Input: part model. Units: mm. Frame: model coordinates. A direction names the side the tool comes from. Coordinates: 2 decimals unless noted, no trailing zeros. Loops run counter-clockwise (first coordinate to the right, second up) from the corner with the lowest first, then second, coordinate; pieces in that order, holes last. Notation, with made-up numbers: (-11.5, -4) -> (29.5, -4) arc R14 ccw to (29.5, 9) -> close; hole circle Ø11 at (-16.5, -4). An arc over 180 degrees is marked (long way). Answer as a JSON object with one key per item and string values.
from build123d import *

# Parameters (mm, degrees)
SKETCH1_R           = 2
SKETCH1_R_2         = 4
SKETCH1_R_3         = 1.95
SKETCH1_R_4         = 1.5
BOSS_EXTRUDE1_DEPTH = 3


with BuildPart() as part:
    # Sketch1 → Boss-Extrude1 (new body)
    with BuildSketch(Plane.XY.offset(-5.551615438)):
        with BuildLine():
            Line((-25.464626351, 10.13731735), (25.464626351, 10.13731735))
            ThreePointArc((25.464626351, 10.13731735), (26.878839913, 9.551530913), (27.464626351, 8.13731735))
            Line((27.464626351, 8.13731735), (27.464626351, -6.86268265))
            ThreePointArc((27.464626351, -6.86268265), (26.878839913, -8.276896212), (25.464626351, -8.86268265))
            Line((25.464626351, -8.86268265), (10, -8.86268265))
            Line((10, -8.86268265), (10, -24.66268265))
            Line((10, -24.66268265), (7.1, -24.66268265))
            Line((7.1, -24.66268265), (7.1, -20.66268265))
            Line((7.1, -20.66268265), (8.4, -20.66268265))
            Line((8.4, -20.66268265), (8.4, -17.86268265))
            Line((8.4, -17.86268265), (7.1, -17.86268265))
            Line((7.1, -17.86268265), (7.1, -6.86268265))
            Line((7.1, -6.86268265), (2.9, -6.86268265))
            Line((2.9, -6.86268265), (2.9, -17.86268265))
            Line((2.9, -17.86268265), (1.6, -17.86268265))
            Line((1.6, -17.86268265), (1.6, -20.66268265))
            Line((1.6, -20.66268265), (2.9, -20.66268265))
            Line((2.9, -20.66268265), (2.9, -24.66268265))
            Line((2.9, -24.66268265), (0, -24.66268265))
            Line((0, -24.66268265), (-2.9, -24.66268265))
            Line((-2.9, -24.66268265), (-2.9, -20.66268265))
            Line((-2.9, -20.66268265), (-1.6, -20.66268265))
            Line((-1.6, -20.66268265), (-1.6, -17.86268265))
            Line((-1.6, -17.86268265), (-2.9, -17.86268265))
            Line((-2.9, -17.86268265), (-2.9, -6.86268265))
            Line((-2.9, -6.86268265), (-7.1, -6.86268265))
            Line((-7.1, -6.86268265), (-7.1, -17.86268265))
            Line((-7.1, -17.86268265), (-8.4, -17.86268265))
            Line((-8.4, -17.86268265), (-8.4, -20.66268265))
            Line((-8.4, -20.66268265), (-7.1, -20.66268265))
            Line((-7.1, -20.66268265), (-7.1, -24.66268265))
            Line((-7.1, -24.66268265), (-10, -24.66268265))
            Line((-10, -24.66268265), (-10, -8.86268265))
            Line((-10, -8.86268265), (-25.464626351, -8.86268265))
            ThreePointArc((-25.464626351, -8.86268265), (-26.878839913, -8.276896212), (-27.464626351, -6.86268265))
            Line((-27.464626351, -6.86268265), (-27.464626351, 8.13731735))
            ThreePointArc((-27.464626351, 8.13731735), (-26.878839913, 9.551530913), (-25.464626351, 10.13731735))
        make_face()
        with Locations((-24.464626351, 5.63731735)):
            Circle(SKETCH1_R, mode=Mode.SUBTRACT)
        with Locations((-24.464626351, -4.36268265)):
            Circle(SKETCH1_R, mode=Mode.SUBTRACT)
        with Locations((23.535373649, -4.36268265)):
            Circle(SKETCH1_R, mode=Mode.SUBTRACT)
        with Locations((23.535373649, 5.63731735)):
            Circle(SKETCH1_R, mode=Mode.SUBTRACT)
        with Locations((9.535373649, 0.63731735)):
            Circle(SKETCH1_R_2, mode=Mode.SUBTRACT)
        with Locations((-10.464626351, 0.63731735)):
            Circle(SKETCH1_R_3, mode=Mode.SUBTRACT)
        with Locations((-24.464626351, 0.63731735)):
            Circle(SKETCH1_R_4, mode=Mode.SUBTRACT)
        with Locations((23.535373649, 0.63731735)):
            Circle(SKETCH1_R_4, mode=Mode.SUBTRACT)
    extrude(amount=BOSS_EXTRUDE1_DEPTH)


solid = part.part
1. Line query: line 1 along X through (y, z) = (-12, -3.4); line 2 along X through (y, z) = (-18.5, -3.9); line 3 along Y through (x, z) = (-2, -2.8). Output: solid intervals per line, ascending.
Reply:
{"line 1": "x = -10 to -7.1, -2.9 to 2.9, 7.1 to 10", "line 2": "x = -10 to -8.4, -1.6 to 1.6, 8.4 to 10", "line 3": "y = -24.66 to -20.66, -17.86 to 10.14"}
2. Section query C-C (x = -11.5). Return loops of the section in (y, z), plus the area to 3 significant figures.
Reply:
{"outline": "(-8.86, -5.55) -> (-1.02, -5.55) -> (-1.02, -2.55) -> (-8.86, -2.55) -> close; (2.29, -5.55) -> (10.14, -5.55) -> (10.14, -2.55) -> (2.29, -2.55) -> close", "area": "47.1 mm2"}
3. Section query A-A (y = -10.5). Return loops of the section in (x, z), plus the area to 3 significant figures.
Reply:
{"outline": "(-10, -5.55) -> (-7.1, -5.55) -> (-7.1, -2.55) -> (-10, -2.55) -> close; (-2.9, -5.55) -> (2.9, -5.55) -> (2.9, -2.55) -> (-2.9, -2.55) -> close; (7.1, -5.55) -> (10, -5.55) -> (10, -2.55) -> (7.1, -2.55) -> close", "area": "34.8 mm2"}
4. Mould query, pull axis X, two halves, no side actions, for faces 5 (the face through (27.465, 1, -4)), 6 (the face through (-9, -24.663, -4)), 7 (the face through (8.4, -19, -4)), 8 (the face through (-1.6, -19, -4)). Classes: pulls with the +X half, pulls with the -X half, needs draft (parallel to the pull), parting line crosses it, or undercut.
Reply:
{"face 5": "pulls with the +X half", "face 6": "needs draft", "face 7": "undercut", "face 8": "undercut"}
5. Access query for faces 1 (the face through (10, -17, -4)), 2 (the face through (-8, -17.863, -4)), 3 (the face through (0, 10.137, -4)), 4 (the face through (2.9, -23, -4)). Directions: +Z, -Z, +X, -X, +Y, -Y. A direction counts if a zero-diameter tool reaches every point of the face in a straight line with its end or side. Return the directions, or none.
Reply:
{"face 1": "+Z, -Z, +X, -Y", "face 2": "+Z, -Z", "face 3": "+Z, -Z, +X, -X, +Y", "face 4": "+Z, -Z, -Y"}
6. Section query B-B (x = 12). Return loops of the section in (y, z), plus the area to 3 significant figures.
Reply:
{"outline": "(-8.86, -5.55) -> (-2.51, -5.55) -> (-2.51, -2.55) -> (-8.86, -2.55) -> close; (3.79, -5.55) -> (10.14, -5.55) -> (10.14, -2.55) -> (3.79, -2.55) -> close", "area": "38.1 mm2"}
7. Pin query (flat end, axial travel): P1, Ø10.5, axis at x = 9.54, y = 0.64, coming from the +Z side; P2, Ø0.9, axis at y = -10, z = -4.5, coming from the +X side; P3, Ø1.5, axis at y = -12, z = -3.5, coming from the -X side; P4, Ø1.5, axis at x = 20.5, z = -4, coming from the -Y side. Return the tip coordinate at first contact, or that it passes through.
Reply:
{"P1": "stops at z = -2.55", "P2": "stops at x = 10", "P3": "stops at x = -10", "P4": "stops at y = -8.86"}
8. Section query D-D (z = -3.05). Count the separate pieces of the cut face and the enclosed holes in it, plus the area to 3 significant figures.
Reply:
{"separate pieces": "1", "enclosed holes": "8", "area": "1,070 mm2"}
